Verification items for the finished model (mm, model axes). A direction names the side the tool comes from. Round coordinates to 2 decimals unless told otherwise and drop trailing zeros. Order: outer loops, then holes, each group sorted by start corner. A loop starts at its lowest first (then second) coordinate and runs counter-clockwise, first axis right, second up. Notation, with made-up numbers: (70, 70) -> (112, 70) arc R29 cw to (112, 100) -> close; hole circle Ø5 at (-3.75, 8.25). An arc over 180 degrees is marked (long way). Return JSON: item names as keys, results as strings. Group by question number.
Item 1: Sectioned sample at B-B on x = -16.5. Record the cut outline in (y, z).
Item 2: Scan lines: probe 1 along Z at (x, y) = (-28, 11); probe 2 along Z at (x, y) = (-3.5, -0.25) (3 decimals); probe 3 along Z at (x, y) = (-7, 5.25). Record each from-to range of solid material in increasing order. Write a range as from..to.
Item 3: Draft check along X on faces 4 (the flat face through (-3.4, -2, -7)), 5 (the flat face through (-37, 8, -148)). Enter one of: pulls with the +X half, pulls with the -X half, needs draft (parallel to the pull), parting line crosses it, or undercut.
Item 4: Access from +Z, -Z, +X, -X, +Y, -Y to the whole of each face (thin tool, end or side, straight path). Record for faces 1 (the flat face through (-18, -1, -94)), 2 (the flat face through (-64, 15, -36)), 3 (the cylindrical face through (-8.627, 7.395, -8.247)).
Item 5: Depth check by flat-ended pin: pin 1 Ø0.9 at (x, y) = (-65.5, -3) entering from +Z; pin 2 Ø8.5 at (x, z) = (-65, -8.5) entering from +Y; pin 3 Ø3.5 at (x, z) = (-65.5, -6) entering from -Y. Enter the tip coordinate at first touch or a pass-through.
Item 6: Sectioned sample at C-C on x = -56.5. Record the cut outline in (y, z), plus the area to 3 significant figures.
Item 7: Sectioned sample at D-D on z = -123. Record the cut outline in (x, y).
Autodesk Inventor part; units mm, degrees
ref_plane "YZ Plane" through (0, 0, 0) normal (1, 0, 0) x (0, 1, 0)
ref_plane "XZ Plane" through (0, 0, 0) normal (0, 1, 0) x (-1, 0, 0)
ref_plane "XY Plane" through (0, 0, 0) normal (0, 0, 1) x (1, 0, 0)
sketch "Sketch1" plane through (0, 0, 0) normal (0, 1, 0) x (-1, 0, 0)
  line L0 (0, 0) -> (73, 0)
  line L1 (73, 0) -> (73, -148)
  line L2 (73, -148) -> (0, -148)
  line L3 (0, -148) -> (0, 0)
  dimension "d0" = 73
  dimension "d1" = 148
extrude "Extrusion1" add sketch "Sketch1" against normal blind 4
sketch "Sketch2" plane through (0, 0, 0) normal (0, 1, 0) x (1, 0, 0)
  line L0 (-73, 148) -> (0, 148)
  line L1 (0, 148) -> (0, 0)
  line L2 (0, 148) -> (0, 0)
  line L3 (0, 0) -> (-73, 0)
  line L4 (0, 0) -> (-73, 0)
  line L5 (-73, 0) -> (-73, 148)
  line L6 (0, 148) -> (0, 144) construction
  line L7 (0, 148) -> (0, 0) construction
  line L8 (0, 144) -> (-4, 144) construction
  line L9 (-4, 144) -> (-69, 144)
  line L10 (-69, 144) -> (-69, 4)
  line L11 (-69, 4) -> (-4, 4)
  line L12 (-4, 4) -> (-4, 144)
  dimension "d4" = 4
  dimension "d5" = 4
  dimension "d6" = 90
  dimension "d7" = 65
  dimension "d8" = 140
extrude "Extrusion2" add sketch "Sketch2" along normal blind 18
sketch "Sketch4" plane through (0, 0, 0) normal (0, 1, 0) x (1, 0, 0)
  line L0 (-4, 4) -> (-4, 144)
  line L1 (-4, 4) -> (-10, 4)
  line L2 (-10, 4) -> (-10, 10)
  line L3 (-10, 10) -> (-4, 10)
  line L4 (-4, 10) -> (-4, 4)
  point P0 (0, 0)
  dimension "d17" = 6
  dimension "d18" = 6
extrude "Extrusion4" add sketch "Sketch4" along normal blind 15
sketch "Sketch9" plane through (0, -4, 0) normal (0, -1, 0) x (1, 0, 0)
  line L0 (0, 0) -> (0, -148) construction
  line L1 (0, 0) -> (-7, 0) construction
  line L2 (0, 0) -> (-73, 0) construction
  line L3 (-7, 0) -> (-7, -7) construction
  circle A0 centre (-7, -7) radius 2.05
  dimension "d60" = 7
  dimension "d61" = 7
  dimension "d62" = 4.1
extrude "Extrusion10" cut sketch "Sketch9" against normal blind 20
sketch "Sketch10" plane through (0, -4, 0) normal (0, -1, 0) x (1, 0, 0)
  circle A0 centre (-7, -7) radius 2.05 construction
  line L0 (-7, -7) -> (-7, 0) construction
  line L1 (0, 0) -> (-73, 0) construction
  line L2 (-7, -7) -> (-10.6, -7) construction
  line L3 (-7, -7) -> (-3.4, -7) construction
  line L4 (-7, -7) -> (-7, -10.875) construction
  line L5 (-7, -7) -> (-7, -3.125) construction
  line L6 (-7, -3.125) -> (-10.6, -3.125)
  line L7 (-10.6, -3.125) -> (-10.6, -10.875)
  line L8 (-10.6, -10.875) -> (-3.4, -10.875)
  line L9 (-3.4, -10.875) -> (-3.4, -3.125)
  line L10 (-3.4, -3.125) -> (-7, -3.125)
  dimension "d65" = 3.6
  dimension "d66" = 3.6
  dimension "d67" = 3.875
  dimension "d68" = 3.875
  dimension "d69" = 7.75
  dimension "d70" = 7.2
extrude "Extrusion11" cut sketch "Sketch10" against normal blind 4
sketch "Sketch11" plane through (0, 0, 0) normal (0, 1, 0) x (1, 0, 0)
  line L0 (-10, 10) -> (-10, 4)
  line L1 (-10, 4) -> (-11.6, 4)
  line L2 (-69, 4) -> (-10, 4)
  line L3 (-11.6, 4) -> (-11.6, 11.6)
  line L4 (-11.6, 4) -> (-4, 4) construction
  line L5 (-11.6, 11.6) -> (-4, 11.6)
  line L6 (-4, 10.875) -> (-4, 144)
  line L7 (-4, 10) -> (-10, 10)
  line L8 (-10, 4) -> (-10, 10)
  line L9 (-10, 10) -> (-4, 10)
  line L10 (-4, 10) -> (-4, 11.6)
  point P0 (0, 0)
  dimension "d73" = 1.6
  dimension "d75" = 90
  dimension "d76" = 1.6
extrude "Extrusion12" add sketch "Sketch11" along normal blind 1.2
pattern_linear "Rectangular Pattern3" count 2 spacing 59 along (-1, 0, 0) count 2 spacing 134 along (0, 0, -1) of "Extrusion4", "Extrusion10", "Extrusion11"
sketch "Sketch12" plane through (0, 0, 0) normal (0, 1, 0) x (1, 0, 0)
  line L0 (-63, 4) -> (-10, 4)
  line L1 (-63, 4) -> (-61.4, 4)
  line L2 (-63, 4) -> (-63, 10)
  line L3 (-63, 4) -> (-63, 10)
  line L4 (-63, 10) -> (-69, 10)
  line L5 (-69, 10) -> (-69, 11.6)
  line L6 (-69, 11.6) -> (-61.4, 11.6)
  line L7 (-61.4, 11.6) -> (-61.4, 4)
  line L8 (-10, 144) -> (-63, 144)
  line L9 (-63, 144) -> (-61.4, 144)
  line L10 (-63, 138) -> (-63, 144)
  line L11 (-63, 144) -> (-63, 138)
  line L12 (-69, 138) -> (-63, 138)
  line L13 (-63, 138) -> (-69, 138)
  line L14 (-69, 138) -> (-69, 136.4)
  line L15 (-69, 137.125) -> (-69, 10.875)
  line L16 (-69, 136.4) -> (-61.4, 136.4)
  line L17 (-61.4, 136.4) -> (-61.4, 144)
  line L18 (-10, 144) -> (-10.6, 144)
  line L19 (-10, 144) -> (-11.6, 144)
  line L20 (-10, 144) -> (-8.4, 144) construction
  line L21 (-10, 144) -> (-10, 138)
  line L22 (-4, 138) -> (-10, 138)
  line L23 (-10, 144) -> (-10, 138)
  line L24 (-10, 138) -> (-4, 138)
  line L25 (-4, 138) -> (-4, 136.4)
  line L26 (-4, 10) -> (-4, 138)
  line L27 (-4, 136.4) -> (-11.6, 136.4)
  line L28 (-11.6, 136.4) -> (-11.6, 144)
  point P0 (0, 0)
  dimension "d85" = 1.6
  dimension "d86" = 1.6
  dimension "d87" = 90
  dimension "d88" = 1.6
  dimension "d89" = 1.6
  dimension "d90" = 90
  dimension "d91" = 1.6
  dimension "d92" = 180
  dimension "d93" = 1.6
  dimension "d94" = 90
extrude "Extrusion13" add sketch "Sketch12" along normal blind 1.2
sketch "Sketch13" plane through (0, 0, 0) normal (0, 1, 0) x (1, 0, 0)
  line L0 (-4, 10) -> (-4, 138) construction
  line L1 (-4, 11.4955) -> (-4, 31.4955) construction
  line L2 (-4, 31.4955) -> (-8, 31.4955) construction
  line L3 (-8, 31.4955) -> (-69, 31.4955) construction
  line L4 (-69, 31.4955) -> (-69, 100.4955) construction
  line L5 (-69, 100.4955) -> (-8, 100.4955) construction
  line L6 (-8, 100.4955) -> (-8, 31.4955) construction
  line L7 (-69, 100.4955) -> (-69, 94.9955) construction
  line L8 (-69, 138) -> (-69, 10) construction
  line L9 (-69, 94.9955) -> (-16.5, 94.9955) construction
  circle A0 centre (-16.5, 94.9955) radius 3.5
  line L10 (-69, 94.9955) -> (-65.5, 94.9955) construction
  circle A1 centre (-65.5, 94.9955) radius 3.5
  line L11 (-65.5, 94.9955) -> (-2, 94.9955) construction
  line L12 (-65.5, 94.9955) -> (-65.5, 36.9955) construction
  circle A2 centre (-65.5, 36.9955) radius 3.5
  line L13 (-69, 31.4955) -> (-11.5, 31.4955) construction
  line L14 (-11.5, 31.4955) -> (-11.5, 36.9955) construction
  circle A3 centre (-11.5, 36.9955) radius 3.5
  circle A4 centre (-65.5, 36.9955) radius 1.55
  circle A5 centre (-16.5, 94.9955) radius 1.55
  circle A6 centre (-11.5, 36.9955) radius 1.55
  circle A7 centre (-65.5, 94.9955) radius 1.55
  point P0 (0, 0)
  dimension "d97" = 20
  dimension "d98" = 4
  dimension "d99" = 61
  dimension "d100" = 69
  dimension "d101" = 5.5
  dimension "d102" = 52.5
  dimension "d103" = 90
  dimension "d104" = 7
  dimension "d105" = 3.5
  dimension "d106" = 7
  dimension "d109" = 58
  dimension "d110" = 7
  dimension "d111" = 57.5
  dimension "d112" = 5.5
  dimension "d113" = 7
  dimension "d114" = 3.1
  dimension "d116" = 3.1
  dimension "d117" = 3.1
  dimension "d118" = 3.1
extrude "Extrusion14" add sketch "Sketch13" along normal blind 15
sketch "Sketch14" plane through (-65.5, 0, -36.9955) normal (0, 1, 0) x (1, 0, 0)
  circle A0 centre (49, 58) radius 1.55
  circle A1 centre (49, 58) radius 1.55
  circle A2 centre (0, 58) radius 1.55
  circle A3 centre (0, 58) radius 1.55
  circle A4 centre (0, 0) radius 1.55
  circle A5 centre (54, 0) radius 1.55
  circle A6 centre (54, 0) radius 1.55
  point P0 (65.5, -36.9955)
  dimension "d121" = 3.1
extrude "Extrusion15" cut sketch "Sketch14" against normal blind 100
sketch "Sketch15" plane through (0, -4, 0) normal (0, -1, 0) x (1, 0, 0)
  circle A0 centre (-11.5, -36.9955) radius 1.55 construction
  line L0 (-11.5, -36.9955) -> (-11.5, -34.1955) construction
  line L1 (-11.5, -34.1955) -> (-14.6, -34.1955) construction
  line L2 (-14.6, -34.1955) -> (-14.6, -39.7955)
  line L3 (-14.6, -39.7955) -> (-8.4, -39.7955)
  line L4 (-14.6, -34.1955) -> (-8.4, -34.1955)
  line L5 (-8.4, -34.1955) -> (-8.4, -39.7955)
  circle A1 centre (-65.5, -36.9955) radius 1.55 construction
  line L6 (-65.5, -36.9955) -> (-62.4, -36.9955) construction
  line L7 (-62.4, -36.9955) -> (-62.4, -39.7955) construction
  line L8 (-62.4, -39.7955) -> (-68.6, -39.7955)
  line L9 (-68.6, -39.7955) -> (-68.6, -34.1955)
  line L10 (-68.6, -34.1955) -> (-62.4, -34.1955)
  line L11 (-62.4, -34.1955) -> (-62.4, -39.7955)
  circle A2 centre (-16.5, -94.9955) radius 1.55 construction
  line L12 (-16.5, -94.9955) -> (-16.5, -97.7955) construction
  line L13 (-16.5, -97.7955) -> (-13.4, -97.7955) construction
  line L14 (-13.4, -97.7955) -> (-19.6, -97.7955)
  line L15 (-19.6, -97.7955) -> (-19.6, -92.1955)
  line L16 (-19.6, -92.1955) -> (-13.4, -92.1955)
  line L17 (-13.4, -92.1955) -> (-13.4, -97.7955)
  line L18 (-65.5, -94.9955) -> (-65.5, -97.7955) construction
  line L19 (-65.5, -97.7955) -> (-62.4, -97.7955) construction
  line L20 (-62.4, -97.7955) -> (-68.6, -97.7955)
  line L21 (-68.6, -97.7955) -> (-68.6, -92.1955)
  line L22 (-68.6, -92.1955) -> (-62.4, -92.1955)
  line L23 (-62.4, -92.1955) -> (-62.4, -97.7955)
  point P0 (0, 0)
  dimension "d124" = 2.8
  dimension "d125" = 3.1
  dimension "d126" = 5.6
  dimension "d127" = 6.2
  dimension "d130" = 3.1
  dimension "d131" = 2.8
  dimension "d132" = 6.2
  dimension "d133" = 5.6
  dimension "d134" = 2.8
  dimension "d135" = 3.1
  dimension "d136" = 6.2
  dimension "d137" = 5.6
  dimension "d138" = 2.8
  dimension "d139" = 3.1
  dimension "d140" = 6.2
  dimension "d141" = 5.6
extrude "Extrusion17" cut sketch "Sketch15" against normal blind 3
sketch "Sketch17" plane through (0, 18, 0) normal (0, 1, 0) x (1, 0, 0)
  line L0 (-69, 4) -> (-69, 144)
  line L1 (-4, 144) -> (-4, 4)
  line L2 (-69, 144) -> (-4, 144)
  line L3 (-4, 144) -> (-4, 4)
  line L4 (-4, 4) -> (-69, 4)
  line L5 (-69, 4) -> (-69, 144)
  line L6 (-4, 4) -> (-5.9, 4) construction
  line L7 (-5.9, 4) -> (-5.9, 2.1828) construction
  line L8 (-5.9, 2.1828) -> (-4, 2.1828) construction
  line L9 (-4, 2.1828) -> (-4, 4) construction
  line L10 (-4, 4) -> (-1.9, 4) construction
  line L11 (-1.9, 4) -> (-1.9, 1.9) construction
  line L12 (-69, 144) -> (-71.1, 144) construction
  line L13 (-71.1, 144) -> (-71.1, 146.1) construction
  line L14 (-71.1, 146.1) -> (-1.9, 146.1)
  line L15 (-1.9, 146.1) -> (-1.9, 1.9)
  line L16 (-1.9, 1.9) -> (-71.1, 1.9)
  line L17 (-71.1, 1.9) -> (-71.1, 146.1)
  point P0 (0, 0)
  dimension "d144" = 1.9
  dimension "d145" = 2.1
  dimension "d146" = 2.1
  dimension "d147" = 2.1
  dimension "d148" = 2.1
extrude "Extrusion18" cut sketch "Sketch17" against normal blind 4
chamfer "Chamfer1" distance 2 angle 45 8 edges at (-36.5, -4, 0) (-73, 7, 0) (-73, -4, -74) (0, 7, 0) (0, -4, -74) (0, 7, -148) (-36.5, -4, -148) (-73, 7, -148)
properties part number "mangOH bottom"
Recorded:
{
 "1": {"outline": "(-4, -146) -> (-2, -148) -> (18, -148) -> (18, -146.1) -> (14, -146.1) -> (14, -144) -> (0, -144) -> (0, -98.5) -> (15, -98.5) -> (15, -96.55) -> (-1, -96.55) -> (-1, -97.8) -> (-4, -97.8) -> close; (-4, -92.2) -> (-1, -92.2) -> (-1, -93.45) -> (15, -93.45) -> (15, -91.5) -> (0, -91.5) -> (0, -4) -> (14, -4) -> (14, -1.9) -> (18, -1.9) -> (18, 0) -> (-2, 0) -> (-4, -2) -> close"},
 "2": {"probe 1": "-148..-144, -4..0", "probe 2": "-148..-144.875, -137.125..-10.875, -3.125..0", "probe 3": "-148..-143.05, -138.95..-138, -10..-9.05, -4.95..0"},
 "3": {"face 4": "undercut", "face 5": "needs draft"},
 "4": {"face 1": "-Y", "face 2": "+Y", "face 3": "+Y, -Y"},
 "5": {"pin 1": "z = -0.55", "pin 2": "y = 15", "pin 3": "y = 0"},
 "6": {"outline": "(-4, -146) -> (-2, -148) -> (18, -148) -> (18, -146.1) -> (14, -146.1) -> (14, -144) -> (0, -144) -> (0, -4) -> (14, -4) -> (14, -1.9) -> (18, -1.9) -> (18, 0) -> (-2, 0) -> (-4, -2) -> close", "area": "715 mm²"},
 "7": {"outline": "(-73, -2) -> (-71, -4) -> (-2, -4) -> (0, -2) -> (0, 18) -> (-1.9, 18) -> (-1.9, 14) -> (-4, 14) -> (-4, 0) -> (-69, 0) -> (-69, 14) -> (-71.1, 14) -> (-71.1, 18) -> (-73, 18) -> close"}
}
